from build123d import *

# Parameters (mm, degrees)
SKETCH1_W           = 10.16
SKETCH1_H           = 10.16
BOSS_EXTRUDE1_DEPTH = 2.54
SKETCH2_W           = 10.16
SKETCH2_H           = 2.54
BOSS_EXTRUDE2_DEPTH = 7.62
SKETCH3_R           = 1.397
CUT_EXTRUDE1_DEPTH  = 10.16
SKETCH4_R           = 1.397
CUT_EXTRUDE2_DEPTH  = 10.16


with BuildPart() as part:
    # Sketch1 → Boss-Extrude1 (new body)
    with BuildSketch(Plane.XY):
        with Locations((5.08, 5.08)):
            Rectangle(SKETCH1_W, SKETCH1_H)
    extrude(amount=BOSS_EXTRUDE1_DEPTH)

    # Sketch2 → Boss-Extrude2 (add)
    with BuildSketch(Plane.XY.offset(2.54)):
        with Locations((5.08, 1.27)):
            Rectangle(SKETCH2_W, SKETCH2_H)
    extrude(amount=BOSS_EXTRUDE2_DEPTH)

    # Sketch3 → Cut-Extrude1 (cut)
    with BuildSketch(Plane.XY.offset(2.54)):
        with Locations((5.08, 6.35)):
            Circle(SKETCH3_R)
    extrude(amount=-CUT_EXTRUDE1_DEPTH, mode=Mode.SUBTRACT)

    # Sketch4 → Cut-Extrude2 (cut)
    with BuildSketch(Plane(origin=(0, 2.54, 0), x_dir=(1, 0, 0), z_dir=(0, 1, 0))):
        with Locations((5.08, -6.35)):
            Circle(SKETCH4_R)
    extrude(amount=-CUT_EXTRUDE2_DEPTH, mode=Mode.SUBTRACT)


solid = part.part
Source: CAD feature listing. Evaluate the final solid. Frame: model axes, mm. A direction names the side the tool comes from. Coordinates: 2 decimals unless noted, no trailing zeros. Loops run counter-clockwise (first coordinate to the right, second up) from the corner with the lowest first, then second, coordinate; pieces in that order, holes last. Notation, with made-up numbers: (-20, 13) - (30, 13) arc R16 cw to (30, 43) - close; hole circle Ø4 at (55, -24). An arc over 180 degrees is marked (long way). One line per question, with ' | ' between items.
1) Line query: line 1 along Z through (x, y) = (5, 2.5); line 2 along X through (y, z) = (0.5, 6.35); line 3 along Y through (x, z) = (5.08, 1.2). Output: solid intervals per line, ascending.
Report:
line 1: z = 0 to 4.96, 7.74 to 10.16 | line 2: x = 0 to 3.68, 6.48 to 10.16 | line 3: y = 0 to 4.95, 7.75 to 10.16
2) First-contact query: P1, Ø1.5, axis at x = 8, z = 5, coming from the +Y side; P2, Ø1.7, axis at x = 5.08, z = 6.35, coming from the -Y side; P3, Ø2.5, axis at x = 5, y = 6, coming from the +Z side. Flat tips, straight axial feed; report the tip coordinate or a pass-through.
Report:
P1: stops at y = 2.54 | P2: passes through | P3: stops at z = 2.54
3) Set-up query: faces 4 (the face through (5, 10.16, 1)), 5 (the face through (4, 2.54, 5)). Return all of +Z, -Z, +X, -X, +Y, -Y with unobstructed straight access to the full face (end or side cutting, diameter ignored); none if empty.
Report:
face 4: +Z, -Z, +X, -X, +Y | face 5: +Z, +X, -X, +Y
4) Section C-C, the plane x = 5.08. Return loops of the section in (y, z), then the cut area to 3 significant figures.
Report:
outline: (0, 0) - (4.95, 0) - (4.95, 2.54) - (2.54, 2.54) - (2.54, 4.95) - (0, 4.95) - close; (0, 7.75) - (2.54, 7.75) - (2.54, 10.16) - (0, 10.16) - close; (7.75, 0) - (10.16, 0) - (10.16, 2.54) - (7.75, 2.54) - close | area: 31.0 mm²
5) Section D-D, the plane z = 2. Return loops of the section in (x, y).
Report:
outline: (0, 0) - (10.16, 0) - (10.16, 10.16) - (0, 10.16) - close; hole circle Ø2.79 at (5.08, 6.35)
6) Section A-A, the plane y = 6.35. Return loops of the section in (x, z), then the cut area to 3 significant figures.
Report:
outline: (0, 0) - (3.68, 0) - (3.68, 2.54) - (0, 2.54) - close; (6.48, 0) - (10.16, 0) - (10.16, 2.54) - (6.48, 2.54) - close | area: 18.7 mm²
7) Pull-direction query (X, two-part tool) for faces 1 (the face through (5, 8, 2.54)), 2 (the face through (0, 3, 2)), 3 (the face through (4.05, 7.294, 1.288)); classes: released by +X, released by -X, zero draft, split by the parting line, or undercut.
Report:
face 1: zero draft | face 2: released by -X | face 3: undercut
